```python
from build123d import *

# Parameters (mm, degrees)
SKETCH1_R           = 4.762499999999989
SKETCH1_R_2         = 4.762500000000005
BOSS_EXTRUDE1_DEPTH = 9.525
CHAMFER1_SIZE       = 88.89999999999999
CHAMFER1_SIZE2      = 6.20588556630559
CHAMFER2_SIZE       = 88.89999999999999
CHAMFER2_SIZE2      = 6.300746042301969
FILLET1_R           = 8.528649
CUT_EXTRUDE2_DEPTH  = 117.6635246642072
FILLET4_R           = 3.175
FILLET5_R           = 12.7
FILLET6_R           = 12.7
SKETCH15_R          = 4.762499999999997
CUT_EXTRUDE7_DEPTH  = 117.28166143642893
FILLET9_R           = 12.7
CUT_EXTRUDE8_DEPTH  = 15.760091062
CUT_EXTRUDE9_DEPTH  = 11.924211795


with BuildPart() as part:
    # Sketch1 → Boss-Extrude1 (new body)
    # profile 1 of 3: a face of its own
    with BuildSketch(Plane.XY):
        Polygon((-28.50000000000001, 23.36447913627793), (-28.500000000000007, 17.01447913627793), (-1.421e-14, 17.01447913627793), (-1.388e-14, 36.06447913627791), (-25.877441230163292, 36.06447913627793), align=None)
        with Locations(Location((-12.700000000000017, 26.539479136277926, 0), (0, 0, 180))):
            Circle(SKETCH1_R, mode=Mode.SUBTRACT)
    # profile 2 of 3: a face of its own
    with BuildSketch(Plane.XY):
        Polygon((1.421e-14, -11.046434023496033), (-28.499999999999996, -11.046434023496033), (-28.499999999999996, -17.396434023496035), (-25.877441230163278, -30.09643402349603), (1.421e-14, -30.09643402349603), align=None)
        with Locations(Location((-12.699999999999989, -20.571434023496032, 0), (0, 0, 180))):
            Circle(SKETCH1_R_2, mode=Mode.SUBTRACT)
    # profile 3 of 3: a face of its own
    with BuildSketch(Plane.XY):
        Polygon((-28.500000000000007, 17.01447913627793), (-28.5, -11.046434023496033), (1.421e-14, -11.046434023496033), (-5.89e-15, 17.014479136277927), align=None)
    extrude(amount=BOSS_EXTRUDE1_DEPTH)

    # Sweep1: sweep along a path in Sketch4
    with BuildLine(Plane(origin=(0, -11.046434023496033, 0), x_dir=(1, 0, 0), z_dir=(0, 1, 0))) as sweep1_path:
        Line((-14.249999999999991, -9.525), (-5.144041152540681, -93.4757286489478))
        Line((-5.144041152540681, -93.4757286489478), (-3.7745316583277084, -106.10167193035296))
    # Sketch3 → Sweep1 (sweep)
    with BuildSketch(Plane.XY.offset(9.525)):
        Polygon((-28.499999999999996, -11.046434023496033), (1.388e-14, -11.046434023496033), (-1.388e-14, 17.01447913627793), (-28.50000000000001, 17.01447913627793), align=None)
    sweep(path=sweep1_path.line)

    # Chamfer1
    chamfer1_edges = [part.edges().sort_by_distance(p)[0] for p in [
        (10.475468341672286, 2.9840225563909506, 106.10167193035296),
    ]]
    chamfer1_side = [part.faces().sort_by_distance(p)[0] for p in [
        (5.237734170836156, 2.9840225563909497, 57.813335965176485),
    ]]
    chamfer(chamfer1_edges, length=CHAMFER1_SIZE, length2=CHAMFER1_SIZE2, reference=chamfer1_side[0])

    # Chamfer2
    chamfer2_edges = [part.edges().sort_by_distance(p)[0] for p in [
        (-18.02453165832772, 2.984022556390949, 106.10167193035296),
    ]]
    chamfer2_side = [part.faces().sort_by_distance(p)[0] for p in [
        (-23.26226582916385, 2.9840225563909497, 57.813335965176506),
    ]]
    chamfer(chamfer2_edges, length=CHAMFER2_SIZE, length2=CHAMFER2_SIZE2, reference=chamfer2_side[0])

    # Fillet1
    fillet1_edges = [part.edges().sort_by_distance(p)[0] for p in [
        (4.269582775366721, 2.984022556390949, 106.10167193035296),
        (-11.72378561602573, 2.984022556390949, 106.10167193035296),
    ]]
    fillet(fillet1_edges, radius=FILLET1_R)

    # Sketch6 → Cut-Extrude2 (cut, through all)
    with BuildSketch(Plane.ZY.offset(28.500000000000004)):
        Polygon((106.10167193035296, -11.046434023496188), (93.47572864894777, -11.0464340234961), (80.70167193035297, -11.046434023496028), (114.70610576395035, -29.45752993708947), (128.32769329374543, 30.37810454166645), (17.720068960516624, 36.90132837728653), (9.525, 17.01447913627794), (80.70167193035296, 8.003565976503989), (106.10167193035296, 8.003565976503813), align=None)
    extrude(amount=-CUT_EXTRUDE2_DEPTH, mode=Mode.SUBTRACT)

    # Fillet4
    fillet4_edges = [part.edges().sort_by_distance(p)[0] for p in [
        (-14.249999999999995, -11.046434023496033, 9.525),
        (-14.25000000000001, 17.01447913627793, 9.525),
    ]]
    fillet(fillet4_edges, radius=FILLET4_R)

    # Fillet5
    fillet5_edges = [part.edges().sort_by_distance(p)[0] for p in [
        (-28.50000000000001, 23.36447913627793, 4.7625),
    ]]
    fillet(fillet5_edges, radius=FILLET5_R)

    # Fillet6
    fillet6_edges = [part.edges().sort_by_distance(p)[0] for p in [
        (-1.404e-14, 36.06447913627791, 4.7625),
        (-25.877441230163292, 36.06447913627793, 4.7625),
    ]]
    fillet(fillet6_edges, radius=FILLET6_R)

    # Sketch15 → Cut-Extrude7 (cut, through all)
    with BuildSketch(Plane(origin=(-2.72e-15, 8.00356597650455, 5.575e-14), x_dir=(1, 3.4e-16, -6e-17), z_dir=(-3.4e-16, 1, 6.99e-15))):
        with Locations(Location((-5.144041152540378, -93.47572864894777, 0), (0, 0, 270))):
            Circle(SKETCH15_R)
    extrude(amount=-CUT_EXTRUDE7_DEPTH, mode=Mode.SUBTRACT)

    # Fillet9
    fillet9_edges = [part.edges().sort_by_distance(p)[0] for p in [
        (1.404e-14, -30.09643402349603, 4.7625),
        (-25.877441230163278, -30.09643402349603, 4.7625),
        (-28.499999999999996, -17.396434023496035, 4.7625),
    ]]
    fillet(fillet9_edges, radius=FILLET9_R)

    # Sketch17 → Cut-Extrude8 (cut)
    with BuildSketch(Plane(origin=(0, 19.81286883339098, 0), x_dir=(1, 0, 0), z_dir=(0, 1, 0))):
        with BuildLine():
            Line((-23.794838845791546, -21.021241844192982), (-14.252419863558526, -74.10090839762722))
            add(Edge.make_bspline(
                [(-14.252419863558526, -74.10090839762722), (-13.55215795886545, -77.99611237791656), (-9.563905474722917, -77.99611237791653)],
                knots=[0.17649604429034987, 0.17649604429034987, 0.17649604429034987, 1.5707963267949046, 1.5707963267949046, 1.5707963267949046], degree=2, weights=[1, 0.7666750083054215, 1]))
            Line((-9.563905474722917, -77.99611237791653), (-4.929711575818474, -77.99611237791652))
            add(Edge.make_bspline(
                [(-4.929711575818474, -77.99611237791652), (0.01696199328928838, -77.99611237791657), (-0.17063766624835885, -73.09214006513507)],
                knots=[1.5707963267948917, 1.5707963267948917, 1.5707963267948917, 3.179526156898573, 3.179526156898573, 3.179526156898573], degree=2, weights=[1, 0.693568883905337, 1]))
            Line((-0.17063766624835885, -73.09214006513507), (-2.201180813451869, -20.012473511700826))
            add(Edge.make_bspline(
                [(-2.201180813451869, -20.012473511700826), (-2.3750711783370813, -15.466870726714172), (-6.960254723021984, -15.466870726714202)],
                knots=[0.03793350330876585, 0.03793350330876585, 0.03793350330876585, 1.5707963267949063, 1.5707963267949063, 1.5707963267949063], degree=2, weights=[1, 0.7203903131485674, 1]))
            Line((-6.960254723021984, -15.466870726714202), (-19.10632445695594, -15.466870726714204))
            add(Edge.make_bspline(
                [(-19.10632445695594, -15.466870726714204), (-24.79337820798673, -15.466870726714157), (-23.794838845791546, -21.021241844192982)],
                knots=[1.5707963267948915, 1.5707963267948915, 1.5707963267948915, 3.318088697880159, 3.318088697880159, 3.318088697880159], degree=2, weights=[1, 0.6420353819221085, 1]))
        make_face()
    extrude(amount=-CUT_EXTRUDE8_DEPTH, mode=Mode.SUBTRACT)

    # Sketch18 → Cut-Extrude9 (cut)
    with BuildSketch(Plane.XZ.offset(11.046434023496033)):
        with BuildLine():
            Line((-4.929711575818475, 77.99611237791653), (-9.563905474722917, 77.99611237791653))
            add(Edge.make_bspline(
                [(-9.563905474722917, 77.99611237791653), (-13.55215795886545, 77.99611237791656), (-14.252419863558526, 74.10090839762722)],
                knots=[4.712388980384682, 4.712388980384682, 4.712388980384682, 6.106689262889237, 6.106689262889237, 6.106689262889237], degree=2, weights=[1, 0.7666750083054213, 1]))
            Line((-14.252419863558526, 74.10090839762722), (-23.794838845791546, 21.021241844192982))
            add(Edge.make_bspline(
                [(-23.794838845791546, 21.021241844192982), (-24.79337820798673, 15.466870726714156), (-19.10632445695594, 15.466870726714204)],
                knots=[2.9650966092994273, 2.9650966092994273, 2.9650966092994273, 4.712388980384695, 4.712388980384695, 4.712388980384695], degree=2, weights=[1, 0.6420353819221084, 1]))
            Line((-19.10632445695594, 15.466870726714204), (-6.960254723021985, 15.466870726714204))
            add(Edge.make_bspline(
                [(-6.960254723021985, 15.466870726714204), (-2.3750711783370777, 15.46687072671417), (-2.201180813451869, 20.012473511700826)],
                knots=[4.71238898038468, 4.71238898038468, 4.71238898038468, 6.245251803870821, 6.245251803870821, 6.245251803870821], degree=2, weights=[1, 0.7203903131485672, 1]))
            Line((-2.201180813451869, 20.012473511700826), (-0.17063766624835808, 73.09214006513507))
            add(Edge.make_bspline(
                [(-0.17063766624835808, 73.09214006513507), (0.0169619932892866, 77.99611237791657), (-4.929711575818475, 77.99611237791653)],
                knots=[3.103659150281014, 3.103659150281014, 3.103659150281014, 4.712388980384695, 4.712388980384695, 4.712388980384695], degree=2, weights=[1, 0.693568883905337, 1]))
        make_face()
    extrude(amount=-CUT_EXTRUDE9_DEPTH, mode=Mode.SUBTRACT)


solid = part.part
```
Work out the finished part from the listing and answer in its coordinate system (mm). A direction names the side the tool comes from. Coordinates: 2 decimals unless noted, no trailing zeros. Loops run counter-clockwise (first coordinate to the right, second up) from the corner with the lowest first, then second, coordinate; pieces in that order, holes last.
1) For faces 4 (the cylindrical face through (-13.88, -11.95, 10.48)), 5 (the flat face through (0, 3, 5)), 6 (the flat face through (-18, 26, 9.525)), 7 (the flat face through (-1.4, 8.7, 41)), 8 (the flat face through (-18.957, -5.168, 47.933)), determine the directions among +Z, -Z, +X, -X, +Y, -Y from which every point of the face is accessible in a straight line to the end or side of a thin tool.
Results:
face 4: +Z, +X, -X, -Y
face 5: -Z, +X, +Y, -Y
face 6: +Z, +X, -X, +Y
face 7: +Y
face 8: -Y
2) Flat-ended cylindrical pins translate along their axes: pin 1 (15 mm diameter, centred on x = -5.14, z = 93.48, fed in from +Y); pin 2 (9.5 mm diameter, centred on x = -13.5, y = 11.5, fed in from +Z); pin 3 (1.5 mm diameter, centred on y = 7.5, z = 72.5, fed in from -X); pin 4 (5.5 mm diameter, centred on x = -12.7, y = -20.57, fed in from -Z). Find the tip coordinate at first contact, or state that the pin passes through.
Results:
pin 1: stops at y = 8
pin 2: stops at z = 103.92
pin 3: stops at x = -17.9
pin 4: passes through
3) Section A-A (z = 71) is taken. Give the vertices of the cut face in (x, y), plus the area to 3 significant figures.
Results:
outline: (-18.03, -11.05) - (-14.81, -11.05) - (-14.81, 0.88) - (-0.25, 0.88) - (-0.25, -11.05) - (2.93, -11.05) - (2.93, 9.23) - (-0.25, 9.23) - (-0.25, 4.05) - (-14.81, 4.05) - (-14.81, 9.23) - (-18.03, 9.23) - close
area: 176 mm2
4) For a pull along X with two mould halves and no side action, classify faces 1 (the cylindrical face through (-28.436, -17.372, 4.829)), 2 (the flat face through (-10, 4.053, 46)), 3 (the flat face through (-18, -22, 9.525)) as +X half, -X half, draft (parallel to the pull), parting line (faces both ways), or undercut.
Results:
face 1: -X half
face 2: undercut
face 3: draft
5) Consider probe 1 along Z at (x, y) = (-7.5, 6); probe 2 along Y at (x, z) = (-12, 6); probe 3 along Z at (x, y) = (-20.5, 28.5) (3 decimals). Determine where each line is inside the solid, lowest interval first.
Results:
probe 1: z = 0 to 15.47, 78 to 89.34, 97.61 to 105.59
probe 2: y = -30.08 to -25.28, -15.86 to 21.83, 31.25 to 36.05
probe 3: z = 0 to 9.525
